```python
from build123d import *

# Parameters (mm, degrees)
EXTRUDE_1_DEPTH      = 5.8
SKETCH_2_W           = 11.5
SKETCH_2_H           = 4.8
CUT_EXTRUDE_1_DEPTH  = 6
SKETCH_3_W           = 0.6
SKETCH_3_H           = 0.6
EXTRUDE_2_DEPTH      = 2
EXTRUDE_2_DEPTH_BACK = 6.1
SKETCH_5_W           = 2
SKETCH_5_H           = 4
CUT_EXTRUDE_2_DEPTH  = 1


with BuildPart() as part:
    # 草图1 → 凸台-拉伸1 (new body)
    with BuildSketch(Plane.XY):
        Polygon((4, 0), (4, 0.5), (6, 0.5), (6, 0), (6.5, 0), (6.5, 0.5), (8.5, 0.5), (8.5, 0), (9, 0), (9, 0.5), (11, 0.5), (11, 0), (12.5, 0), (12.5, 7), (0, 7), (0, 0), (1.5, 0), (1.5, 0.5), (3.5, 0.5), (3.5, 0), align=None)
    extrude(amount=EXTRUDE_1_DEPTH)

    # 草图2 → 切除-拉伸1 (cut)
    with BuildSketch(Plane(origin=(0, 7, 0), x_dir=(1, 0, 0), z_dir=(0, 1, 0))):
        with Locations((6.25, -2.9)):
            Rectangle(SKETCH_2_W, SKETCH_2_H)
    extrude(amount=-CUT_EXTRUDE_1_DEPTH, mode=Mode.SUBTRACT)

    # 草图3 → 凸台-拉伸2 (add, two sides)
    with BuildSketch(Plane.XZ) as extrude_2_sk:
        with Locations((5, 3.4)):
            Rectangle(SKETCH_3_W, SKETCH_3_H)
        with Locations((7.5, 3.4)):
            Rectangle(SKETCH_3_W, SKETCH_3_H)
        with Locations((2.5, 3.4)):
            Rectangle(SKETCH_3_W, SKETCH_3_H)
        with Locations((10, 3.4)):
            Rectangle(SKETCH_3_W, SKETCH_3_H)
    extrude(amount=EXTRUDE_2_DEPTH)
    extrude(extrude_2_sk.sketch, amount=-EXTRUDE_2_DEPTH_BACK)

    # 草图5 → 切除-拉伸2 (cut)
    with BuildSketch(Plane.XY.offset(5.8)):
        with Locations((2.5, 5)):
            Rectangle(SKETCH_5_W, SKETCH_5_H)
        with Locations((10, 5)):
            Rectangle(SKETCH_5_W, SKETCH_5_H)
    extrude(amount=-CUT_EXTRUDE_2_DEPTH, mode=Mode.SUBTRACT)


solid = part.part
```
Work out the finished part from the listing and answer in its coordinate system (mm). A direction names the side the tool comes from. Coordinates: 2 decimals unless noted, no trailing zeros. Loops run counter-clockwise (first coordinate to the right, second up) from the corner with the lowest first, then second, coordinate; pieces in that order, holes last. Notation, with made-up numbers: M 39,78 L 94,78 A27 ccw 94,95 Z; hole C 80,9 d2. An arc over 180 degrees is marked long. Use CSV: the item, a comma, the result in double quotes. Start each with the question number.
(1) For faces 1 (the face through (6, 4, 5.8)), 2 (the face through (6, 4, 5.3)), determine the directions among +Z, -Z, +X, -X, +Y, -Y from which every point of the face is accessible in a straight line to the end or side of a thin tool.
(2) Find section D-D, the plane z = 2.55. Give the vertices of the cut face in (x, y), then the cut area to 3 significant figures.
(3) Find section C-C, the plane y = -1. Give the vertices of the cut face in (x, z), then the cut area to 3 significant figures.
(4) Given pin 1 Ø1.5 at (x, z) = (4, 4.5) entering from -Y, flat-ended and moving along its own axis, determine where the tip first touches the part or whether it passes through.
(5) Consider line 1 (X direction, y = 6.75, z = 5.5); line 2 (X direction, y = 3, z = 3.45); line 3 (Z direction, x = 11.5, y = 4). Determine where each line is inside the solid, lowest interval first.
(6) Find section A-A, the plane y = 1.5. Give the vertices of the cut face in (x, z).
(7) Find section B-B, the plane x = 9.25. Give the vertices of the cut face in (y, z).
Recorded:
1,face 1,"+Z, +X, -X, +Y, -Y"
1,face 2,"+Y"
2,outline,"M 0,0 L 1.5,0 L 1.5,0.5 L 3.5,0.5 L 3.5,0 L 4,0 L 4,0.5 L 6,0.5 L 6,0 L 6.5,0 L 6.5,0.5 L 8.5,0.5 L 8.5,0 L 9,0 L 9,0.5 L 11,0.5 L 11,0 L 12.5,0 L 12.5,7 L 12,7 L 12,1 L 0.5,1 L 0.5,7 L 0,7 Z"
2,area,"14.5 mm^2"
3,outline,"M 2.2,3.1 L 2.8,3.1 L 2.8,3.7 L 2.2,3.7 Z; M 4.7,3.1 L 5.3,3.1 L 5.3,3.7 L 4.7,3.7 Z; M 7.2,3.1 L 7.8,3.1 L 7.8,3.7 L 7.2,3.7 Z; M 9.7,3.1 L 10.3,3.1 L 10.3,3.7 L 9.7,3.7 Z"
3,area,"1.44 mm^2"
4,pin 1,"stops at y = 0"
5,line 1,"x = 0 to 1.5, 3.5 to 9, 11 to 12.5"
5,line 2,"x = 0 to 0.5, 2.2 to 2.8, 4.7 to 5.3, 7.2 to 7.8, 9.7 to 10.3, 12 to 12.5"
5,line 3,"z = 0 to 0.5, 5.3 to 5.8"
6,outline,"M 0,0 L 12.5,0 L 12.5,5.8 L 0,5.8 Z; M 2.2,3.1 L 2.8,3.1 L 2.8,3.7 L 2.2,3.7 Z; M 4.7,3.1 L 5.3,3.1 L 5.3,3.7 L 4.7,3.7 Z; M 7.2,3.1 L 7.8,3.1 L 7.8,3.7 L 7.2,3.7 Z; M 9.7,3.1 L 10.3,3.1 L 10.3,3.7 L 9.7,3.7 Z; hole M 0.5,0.5 L 12,0.5 L 12,5.3 L 0.5,5.3 Z"
7,outline,"M 0.5,0 L 7,0 L 7,0.5 L 1,0.5 L 1,5.3 L 3,5.3 L 3,5.8 L 0.5,5.8 Z"
